Drawing for the job (mm, zero at the part's lowest x, y, z). A direction names the side the tool comes from. Coordinates: 2 decimals unless noted, no trailing zeros. Order: outer loops, then holes, each group sorted by start corner. A loop starts at its lowest first (then second) coordinate and runs counter-clockwise, first axis right, second up.
1) Cut at C-C (z = 56.07). List the corners of the cut face in (x, y), and give its area (3 significant figures).
2) Wall check: L1, parallel to Z at x = 8.93, y = 0.3; L2, parallel to Z at x = 31.5, y = 58.5. Give the ranges that are in metal, low to high.
3) Cut at A-A (x = 56.07). List the corners of the cut face in (y, z).
4) Tool access for the marked faces 1 and 2: list every direction of +Z, -Z, +X, -X, +Y, -Y with a clear straight run to the whole face (end or side of a thin tool).
5) Pin check, flat tips, straight feed: pin 1 Ø3 at (x, z) = (52, 28.5) entering from -Y; pin 2 Ø5 at (x, y) = (36, 9.5) entering from -Z; pin 3 Ø6 at (x, z) = (56.07, 56.07) entering from +Y. Stop position of each tip, or through.
6) Cut at B-B (z = 49). List the corners of the cut face in (x, y), and give its area (3 significant figures).
7) Cut at D-D (x = 38). List the corners of the cut face in (y, z), and give its area (3 significant figures).
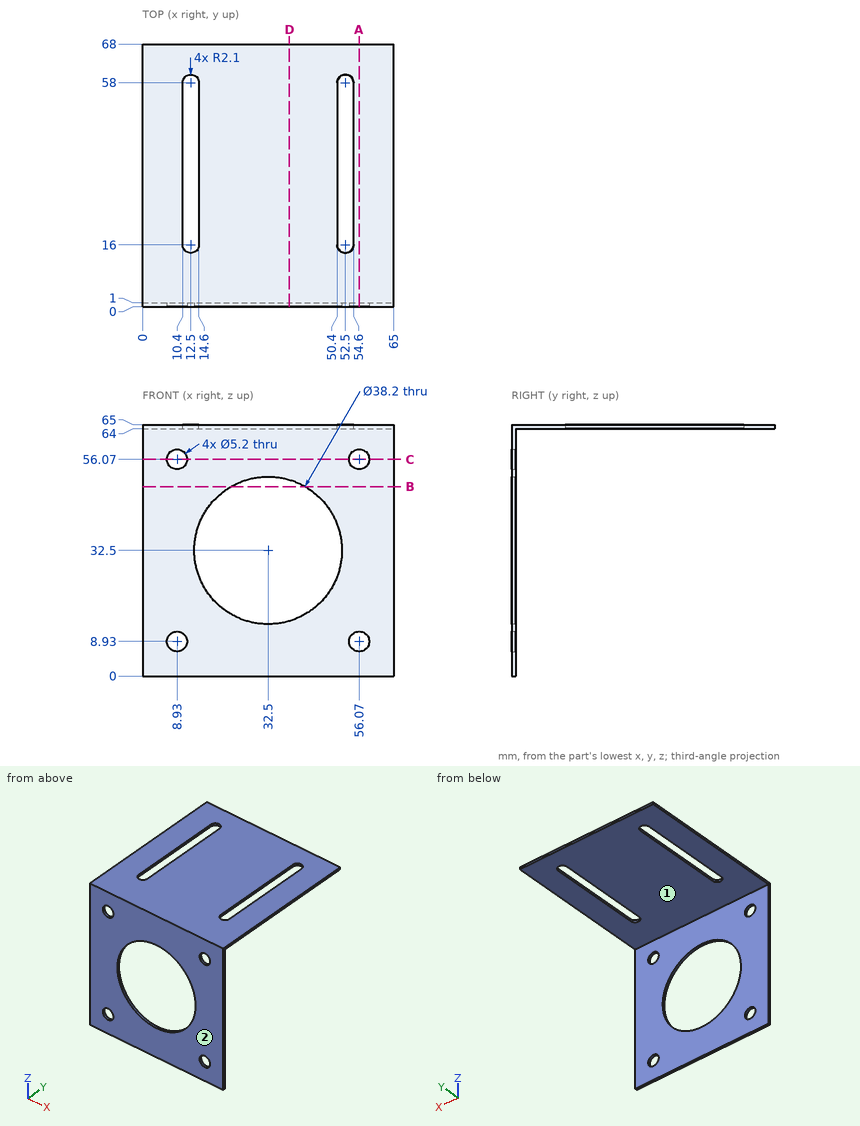
Geometry check:
1. outline: (0, 0) - (6.33, 0) - (6.33, 1) - (0, 1) - close; (11.53, 0) - (53.47, 0) - (53.47, 1) - (11.53, 1) - close; (58.67, 0) - (65, 0) - (65, 1) - (58.67, 1) - close
1. area: 54.6 mm2
2. L1: z = 0 to 6.33, 11.53 to 53.47, 58.67 to 65
2. L2: z = 64 to 65
3. outline: (0, 0) - (1, 0) - (1, 6.33) - (0, 6.33) - close; (0, 11.53) - (1, 11.53) - (1, 53.47) - (0, 53.47) - close; (0, 58.67) - (1, 58.67) - (1, 64) - (68, 64) - (68, 65) - (0, 65) - close
4. face 1: -Z, +X, -X, +Y
4. face 2: +Z, -Z, +X, -X, -Y
5. pin 1: stops at y = 0
5. pin 2: stops at z = 64
5. pin 3: stops at y = 1
6. outline: (0, 0) - (22.88, 0) - (22.88, 1) - (0, 1) - close; (42.12, 0) - (65, 0) - (65, 1) - (42.12, 1) - close
6. area: 45.8 mm2
7. outline: (0, 0) - (1, 0) - (1, 14.21) - (0, 14.21) - close; (0, 50.79) - (1, 50.79) - (1, 64) - (68, 64) - (68, 65) - (0, 65) - close
7. area: 95.4 mm2
